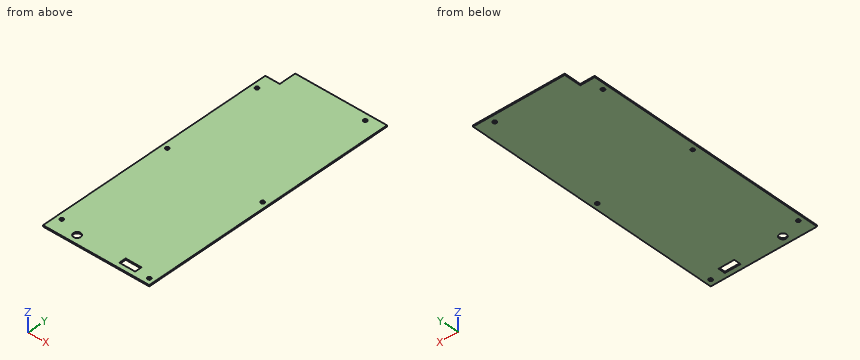
```python
from build123d import *

# Parameters (mm, degrees)
SKETCH3_W              = 88
SKETCH3_H              = 215
BOSS_EXTRUDE3_DEPTH    = 1.1
CUT_EXTRUDE1_OUTLINE_W = 12
CUT_EXTRUDE1_OUTLINE_H = 13.99905087
CUT_EXTRUDE1_OUTLINE_R = 1.5
CUT_EXTRUDE1_DEPTH     = 1.1
SKETCH4_R              = 3
CUT_EXTRUDE2_DEPTH     = 1.1
SKETCH5_W              = 13.1
SKETCH5_H              = 5.72
CUT_EXTRUDE3_DEPTH     = 1.1


# Read off the part's stored shape, not the designer's step: Cut-Extrude1
with BuildPart() as part:
    # Sketch3 → Boss-Extrude3 (new body)
    with BuildSketch(Plane.XY):
        with Locations((0.594511969, -70.924817192)):
            Rectangle(SKETCH3_W, SKETCH3_H)
    extrude(amount=BOSS_EXTRUDE3_DEPTH)

    # Cut-Extrude1 outline → Cut-Extrude1 (cut)
    with BuildSketch(Plane.XY):
        with Locations((-37.405488031, 29.575657373)):
            Rectangle(CUT_EXTRUDE1_OUTLINE_W, CUT_EXTRUDE1_OUTLINE_H)
        with Locations((31.594511969, 31.075182808)):
            Circle(CUT_EXTRUDE1_OUTLINE_R)
        with Locations((-38.905488031, -166.424817192)):
            Circle(CUT_EXTRUDE1_OUTLINE_R)
        with Locations((-38.905488031, -70.924817192)):
            Circle(CUT_EXTRUDE1_OUTLINE_R)
        with Locations((-38.905488031, 10.255182808)):
            Circle(CUT_EXTRUDE1_OUTLINE_R)
        with Locations((40.094511969, -70.924817192)):
            Circle(CUT_EXTRUDE1_OUTLINE_R)
        with Locations((40.094511969, -173.424817192)):
            Circle(CUT_EXTRUDE1_OUTLINE_R)
    extrude(amount=CUT_EXTRUDE1_DEPTH, mode=Mode.SUBTRACT)

    # Sketch4 → Cut-Extrude2 (cut)
    with BuildSketch(Plane.XY.offset(1.1)):
        with Locations((-21.465488031, -171.524817192)):
            Circle(SKETCH4_R)
    extrude(amount=-CUT_EXTRUDE2_DEPTH, mode=Mode.SUBTRACT)

    # Sketch5 → Cut-Extrude3 (cut)
    with BuildSketch(Plane.XY.offset(1.1)):
        with Locations((22.654511969, -171.524817192)):
            Rectangle(SKETCH5_W, SKETCH5_H)
    extrude(amount=-CUT_EXTRUDE3_DEPTH, mode=Mode.SUBTRACT)


solid = part.part
```
Here's how the part is built. I have some questions about the finished solid (model axes, mm). Give positions to 0.01 mm unless a question says otherwise; leave off trailing zeros. Write each loop counter-clockwise with the first axis right and the second up, starting at its lowest first coordinate (ties: lowest second). Pieces come first, ordered by that corner, then holes. Notation, with made-up numbers: M -1.5,-4 L 18.5,-4 A19 cw 18.5,29 Z; hole C 86.25,31.25 d8. An arc over 180 degrees is marked long. Put each result on its own line as item: value. Start each with the question number.
Item 1: If we section it at A-A, the plane x = 27: Write out the boundary of the cut face in (y, z).
Item 2: I need wall thicknesses on L1, parallel to Y at x = 23.5, z = 0.7; L2, parallel to Y at x = -33, z = 0.45; L3, parallel to X at y = 25.5, z = 0.5. Which ranges of each line are inside material? Lowest first, please. Write a range as from..to.
Item 3: If we section it at B-B, the plane z = 0.4: Count the separate pieces of the cut face and the enclosed holes in it, then the cut area to 3 significant figures.
Item 4: Will these pins go through, and if not, where does the flat tip stop? pin 1 (6 mm diameter, centred on x = -14.5, y = -12.5, fed in from -Z); pin 2 (0.6 mm diameter, centred on y = 27, z = 0.5, fed in from -X).
Values:
1. outline: M -178.42,0 L -174.38,0 L -174.38,1.1 L -178.42,1.1 Z; M -168.66,0 L 36.58,0 L 36.58,1.1 L -168.66,1.1 Z
2. L1: -178.42..-174.38, -168.66..36.58
2. L2: -178.42..22.58
2. L3: -31.41..44.59
3. separate pieces: 1
3. enclosed holes: 8
3. area: 18,600 mm²
4. pin 1: z = 0
4. pin 2: x = -31.41
